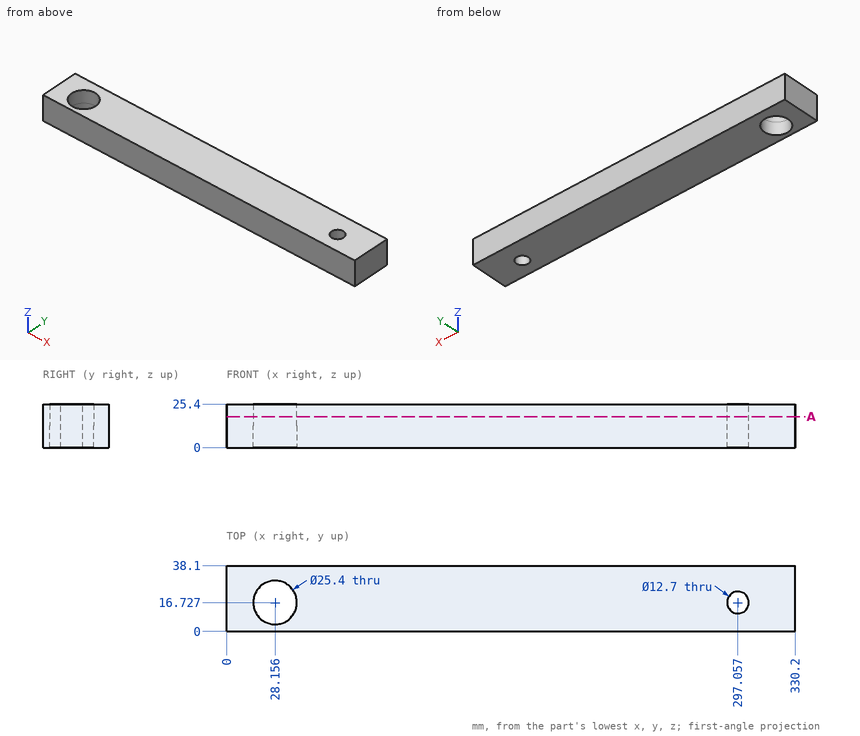
Verification items for this drawing (mm, ordinates from the low corner). Give positions to 0.01 mm unless a question says otherwise; leave off trailing zeros. Write item = value, one per line. Start each with the question number.
Q1. Cross-section at A-A, the plane z = 18. State how many separate pieces and enclosed holes the cut face has, and give its area (3 significant figures).
Q2. Depth check by flat-ended pin: P1, Ø15, axis at x = 28.16, y = 16.73, coming from the +Z side. Enter the tip coordinate at first touch or a pass-through.
Q3. Thickness scan on line 1 (X direction, y = 17, z = 1.25); line 2 (X direction, y = 12, z = 24) (1 decimal); line 3 (X direction, y = 7, z = 23.25). Record the ranges inside material, lowest first.
Answer key:
q1.separate_pieces = 1
q1.enclosed_holes = 2
q1.area = 11,900 mm^2
q2.P1 = through
q3.line_1 = 0 to 15.46, 40.85 to 290.71, 303.4 to 330.2
q3.line_2 = 0 to 16.4, 39.9 to 292.8, 301.3 to 330.2
q3.line_3 = 0 to 19.99, 36.32 to 330.2
